Part model, mm, in its own coordinate system. A direction names the side the tool comes from. Give positions to 0.01 mm unless a question says otherwise; leave off trailing zeros. Write each loop counter-clockwise with the first axis right and the second up, starting at its lowest first coordinate (ties: lowest second). Pieces come first, ordered by that corner, then holes. Notation, with made-up numbers: (18.25, 11.25) - (24.25, 11.25) arc R23 cw to (24.25, 47.25) - close; hole circle Ø2 at (25, 29). An arc over 180 degrees is marked (long way). Answer in a Markdown table with one row per item. Add a question column.
1. Probe line 1 along Y through (x, z) = (69.5, -0.5); line 2 along X through (y, z) = (13, -6.5); line 3 along Z through (x, y) = (37, -16). List the from-to ranges inside material, lowest first.
2. Band-saw the part on C-C on x = 29.5. Write the cut outline in (y, z), plus the area to 3 significant figures.
3. Band-saw the part on A-A on y = 0. Write the cut outline in (x, z).
4. Pull direction X, two halves, no side cores. Call faces 1 (the flat face through (90.5, 7, 10)), 2 (the cylindrical face through (27.115, -4.336, -19.524)), 3 (the cylindrical face through (90.01, -11.99, 0.53)), 4 (the flat face through (55, -9, 9)): released by +X, released by -X, zero draft, split by the parting line, or undercut.
5. Which spindle directions (+Z, -Z, +X, -X, +Y, -Y) get a long thin tool onto all of the face, cutting with end or side? Do faces 5 (the cylindrical face through (102.184, 11.923, 3.755)), 6 (the flat face through (89.5, 7, 10)), 7 (the flat face through (115, 0, 0)). Say none if no direction does.
6. Band-saw the part on D-D on y = -14. Write the cut outline in (x, z), plus the area to 3 significant figures.
7. Drop flat-ended pins along their axis: pin 1 Ø2 at (x, y) = (86.5, 9.5) entering from +Z; pin 2 Ø4 at (x, y) = (23.5, -1.5) entering from +Z; pin 3 Ø4 at (x, y) = (77, 8.5) entering from -Z; pin 4 Ø1 at (x, z) = (81.5, 14) entering from +Y. Give the stop position or say it passes through.
```python
from build123d import *

# Parameters (mm, degrees)
SKIZZE2_W = 1
SKIZZE2_H = 0.5


with BuildPart() as part:
    # Skizze1 → Rotation1 (revolve)
    with BuildSketch(Plane.XY):
        Polygon((0, 20), (0, 0), (115, 0), (115, 11.7), (114.2, 12.5), (55, 12.5), (55, 20), align=None)
    revolve(axis=Axis((0, 0, 0), (1, 0, 0)))

    # Skizze2 → Schnitt-Rotation1 (revolve, cut)
    with BuildSketch(Plane.XY):
        with Locations((90, 12.25)):
            Rectangle(SKIZZE2_W, SKIZZE2_H)
    revolve(axis=Axis((79.835349202, 0, 0), (1, 0, 0)), mode=Mode.SUBTRACT)


solid = part.part
```
Values:
| question | item | result |
|---|---|---|
| 1 | line 1 | y = -12.49 to 12.49 |
| 1 | line 2 | x = 0 to 55 |
| 1 | line 3 | z = -12 to 12 |
| 2 | outline | circle Ø40 at (0, 0) |
| 2 | area | 1,260 mm² |
| 3 | outline | (0, -20) - (55, -20) - (55, -12.5) - (89.5, -12.5) - (89.5, -12) - (90.5, -12) - (90.5, -12.5) - (114.2, -12.5) - (115, -11.7) - (115, 11.7) - (114.2, 12.5) - (90.5, 12.5) - (90.5, 12) - (89.5, 12) - (89.5, 12.5) - (55, 12.5) - (55, 20) - (0, 20) - close |
| 4 | face 1 | undercut |
| 4 | face 2 | zero draft |
| 4 | face 3 | undercut |
| 4 | face 4 | released by +X |
| 5 | face 5 | +X |
| 5 | face 6 | none |
| 5 | face 7 | +Z, -Z, +X, +Y, -Y |
| 6 | outline | (0, -14.28) - (55, -14.28) - (55, 14.28) - (0, 14.28) - close |
| 6 | area | 1,570 mm² |
| 7 | pin 1 | stops at z = 9.17 |
| 7 | pin 2 | stops at z = 20 |
| 7 | pin 3 | stops at z = -10.68 |
| 7 | pin 4 | passes through |
